```python
from build123d import *

# Parameters (mm, degrees)
SKETCH1_W               = 41
SKETCH1_H               = 54
BOSS_EXTRUDE1_DEPTH     = 3
SKETCH2_W               = 41
SKETCH2_H               = 3
BOSS_EXTRUDE2_DEPTH     = 48
SKETCH4_R               = 6
CUT_EXTRUDE1_DEPTH      = 145.103724485
CUT_EXTRUDE3_DEPTH      = 145.103724485
CUT_EXTRUDE3_DEPTH_BACK = 145.103724485
SKETCH12_R              = 6
CUT_EXTRUDE4_DEPTH      = 145.103724485


with BuildPart() as part:
    # Sketch1 → Boss-Extrude1 (new body)
    with BuildSketch(Plane(origin=(0, 0, 0), x_dir=(1, 0, 0), z_dir=(0, 1, 0))):
        with Locations((-104.255294118, -7.041782531)):
            Rectangle(SKETCH1_W, SKETCH1_H)
    extrude(amount=BOSS_EXTRUDE1_DEPTH)

    # Sketch2 → Boss-Extrude2 (add)
    with BuildSketch(Plane(origin=(0, 3, 0), x_dir=(1, 0, 0), z_dir=(0, 1, 0))):
        with Locations((-104.255294118, 18.458217469)):
            Rectangle(SKETCH2_W, SKETCH2_H)
    extrude(amount=BOSS_EXTRUDE2_DEPTH)

    # Sketch4 → Cut-Extrude1 (cut, through all)
    with BuildSketch(Plane.XY.offset(-16.958217469)):
        with Locations((-104.255294118, 37.5)):
            Circle(SKETCH4_R)
    extrude(amount=-CUT_EXTRUDE1_DEPTH, mode=Mode.SUBTRACT)

    # Sketch5 → Cut-Extrude3 (cut, two sides: drawn at the far end of the back side and taken through both)
    with BuildSketch(Plane.XY.offset(-16.958217469).offset(-CUT_EXTRUDE3_DEPTH_BACK)):
        with BuildLine():
            Line((-124.755294118, 51), (-124.755294118, 30.5))
            ThreePointArc((-124.755294118, 30.5), (-118.750983132, 44.995689014), (-104.255294118, 51))
            Line((-104.255294118, 51), (-124.755294118, 51))
        make_face()
        with BuildLine():
            ThreePointArc((-104.255294118, 51), (-89.759605103, 44.995689014), (-83.755294118, 30.5))
            Line((-83.755294118, 30.5), (-83.755294118, 51))
            Line((-83.755294118, 51), (-104.255294118, 51))
        make_face()
    extrude(amount=CUT_EXTRUDE3_DEPTH + CUT_EXTRUDE3_DEPTH_BACK, mode=Mode.SUBTRACT)

    # Sketch12 → Cut-Extrude4 (cut, through all)
    with BuildSketch(Plane.XY.offset(-16.958217469)):
        with Locations((-104.255294118, 16.378845884)):
            Circle(SKETCH12_R)
    extrude(amount=-CUT_EXTRUDE4_DEPTH, mode=Mode.SUBTRACT)


solid = part.part
```
Can you work these out from the model? Positions are in its coordinate system, mm. A direction names the side the tool comes from. Round coordinates to 2 decimals unless told otherwise and drop trailing zeros. Order: outer loops, then holes, each group sorted by start corner. A loop starts at its lowest first (then second) coordinate and runs counter-clockwise, first axis right, second up. Notation, with made-up numbers: (21.25, 86) -> (33.25, 86) arc R9 ccw to (33.25, 90) -> close; hole circle Ø1 at (0, 27.25). An arc over 180 degrees is marked (long way). Return JSON: item names as keys, results as strings. Group by question number.
1. If we section it at D-D, the plane x = -122: Write out the boundary of the cut face in (y, z).
2. I need wall thicknesses on line 1 (Y direction, x = -111.5, z = -5); line 2 (Z direction, x = -122.5, y = 36.5); line 3 (X direction, y = 37, z = -17). Which ranges of each line are inside material? Lowest first, please. Write a range as [from, to].
3. Which directions (+Z, -Z, +X, -X, +Y, -Y) give clear straight access to the entire face, cutting with the end or side of a thin tool? Please do faces 1 (the face through (-124.755, 2.8, 3.2)), 2 (the face through (-105, 27, -16.958)).
4. If we section it at A-A, the plane x = -106.5: Write out the boundary of the cut face in (y, z), then the cut area to 3 significant figures.
5. If we section it at C-C, the plane z = 23: Write out the boundary of the cut face in (x, y), then the cut area to 3 significant figures.
6. We'd pull the mould along Y, two halves only. Please class faces 3 (the face through (-105, 25, -19.958)), 4 (the face through (-98.713, 35.202, -18.437)), 5 (the face through (-105, 0, 7)), 6 (the face through (-105, 3, 8)): released by +Y, released by -Y, zero draft, split by the parting line, or undercut.
7. Will these pins go through, and if not, where does the flat tip stop? pin 1 (1 mm diameter, centred on x = -99.5, z = -3.5, fed in from +Y); pin 2 (6 mm diameter, centred on x = -106.5, y = 7, fed in from +Z); pin 3 (6 mm diameter, centred on y = 40, z = -11, fed in from +X).
8. If we section it at B-B, the plane y = 40.5: Write out the boundary of the cut face in (x, z).
Output values:
{
 "1": {"outline": "(0, -19.96) -> (40.77, -19.96) -> (40.77, -16.96) -> (3, -16.96) -> (3, 34.04) -> (0, 34.04) -> close"},
 "2": {"line 1": "[0, 3]", "line 2": "[-19.96, -16.96]", "line 3": "[-123.7, -110.23], [-98.28, -84.81]"},
 "3": {"face 1": "+Z, -Z, -X, +Y, -Y", "face 2": "+Z, +X, -X, +Y"},
 "4": {"outline": "(0, -19.96) -> (10.81, -19.96) -> (10.81, -16.96) -> (3, -16.96) -> (3, 34.04) -> (0, 34.04) -> close; (21.94, -19.96) -> (31.94, -19.96) -> (31.94, -16.96) -> (21.94, -16.96) -> close; (43.06, -19.96) -> (50.88, -19.96) -> (50.88, -16.96) -> (43.06, -16.96) -> close", "area": "239 mm²"},
 "5": {"outline": "(-124.76, 0) -> (-83.76, 0) -> (-83.76, 3) -> (-124.76, 3) -> close", "area": "123 mm²"},
 "6": {"face 3": "zero draft", "face 4": "undercut", "face 5": "released by -Y", "face 6": "released by +Y"},
 "7": {"pin 1": "y = 3", "pin 2": "z = -16.96", "pin 3": "through"},
 "8": {"outline": "(-122.15, -19.96) -> (-109.45, -19.96) -> (-109.45, -16.96) -> (-122.15, -16.96) -> close; (-99.06, -19.96) -> (-86.36, -19.96) -> (-86.36, -16.96) -> (-99.06, -16.96) -> close"}
}
